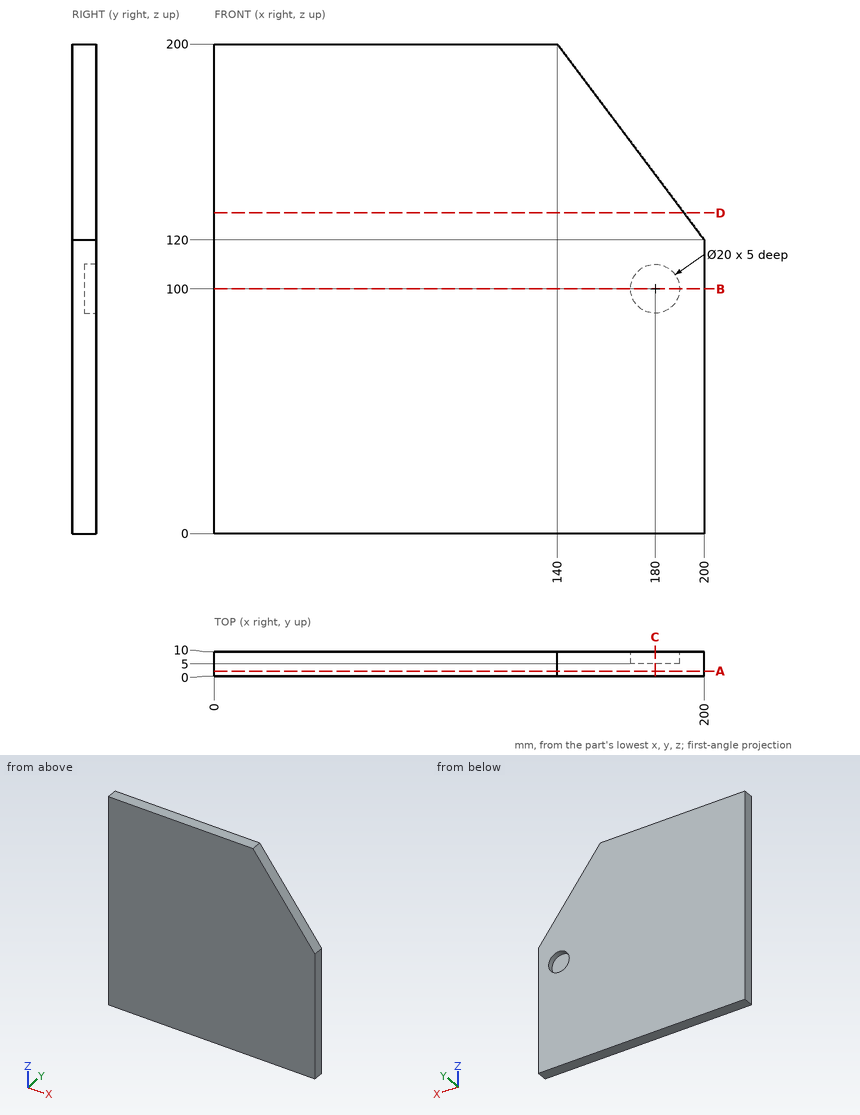
Source: three-view drawing plus pictorial views. Frame: mm from the lowest corner of the part. Round coordinates to 2 decimals unless told otherwise and drop trailing zeros. Loops run counter-clockwise (first coordinate to the right, second up) from the corner with the lowest first, then second, coordinate; pieces in that order, holes last. Notation, with made-up numbers: M 80.5,31 L 93.5,31 A17 ccw 93.5,45 Z; hole C 56.5,41.5 d1. An arc over 180 degrees is marked long. Answer as CSV lines item,"result".
Q1. Cut plane C-C (x = 180). Return the cut outline in (y, z).
Verdict:
outline,"M 0,0 L 10,0 L 10,90 L 5,90 L 5,110 L 10,110 L 10,146.67 L 0,146.67 Z"
Q2. Cut plane A-A (y = 2). Return the cut outline in (x, z).
Verdict:
outline,"M 0,0 L 200,0 L 200,120 L 140,200 L 0,200 Z"
Q3. Line query: line 1 along X through (y, z) = (8.6, 100); line 2 along X through (y, z) = (6.25, 170.5) (3 decimals); line 3 along Z through (x, y) = (162.5, 3). Output: solid intervals per line, ascending.
Verdict:
line 1,"x = 0 to 170, 190 to 200"
line 2,"x = 0 to 162.125"
line 3,"z = 0 to 170"
Q4. Cut plane D-D (z = 131). Return the cut outline in (x, y).
Verdict:
outline,"M 0,0 L 191.75,0 L 191.75,10 L 0,10 Z"
Q5. Cut plane B-B (z = 100). Return the cut outline in (x, y), plus the area to 3 significant figures.
Verdict:
outline,"M 0,0 L 200,0 L 200,10 L 190,10 L 190,5 L 170,5 L 170,10 L 0,10 Z"
area,"1,900 mm^2"
